Geometry: see drawing. Coordinates: mm, zero at the bounding-box minimum. A direction names the side the tool comes from. Give positions to 0.01 mm unless a question says otherwise; leave off trailing zeros. Write each loop counter-clockwise with the first axis right and the second up, starting at its lowest first coordinate (ties: lowest second). Pieces come first, ordered by that corner, then holes. Notation, with made-up numbers: (64, -7) - (79, -7) arc R12 cw to (79, -2) - close; hole circle Ø8 at (26, 41). An arc over 180 degrees is marked (long way). Return JSON: item names as keys, results as strings.
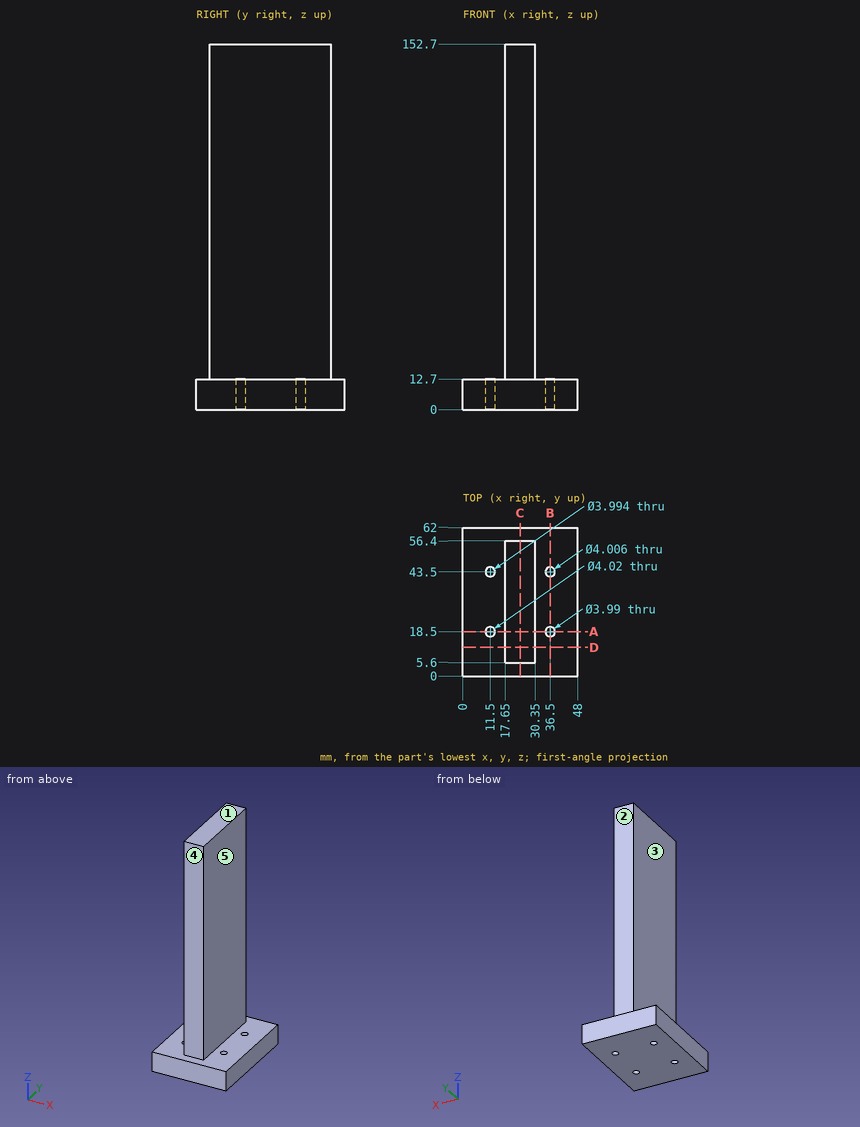
Q1. Set-up query: the marked faces 1, 2, 3, 4 and 5. Return all of +Z, -Z, +X, -X, +Y, -Y with unobstructed straight access to the full face (end or side cutting, diameter ignored); none if empty.
Answer key:
{"face 1": "+Z, +X, -X, +Y, -Y", "face 2": "+Z, +X, -X, +Y", "face 3": "+Z, -X, +Y, -Y", "face 4": "+Z, +X, -X, -Y", "face 5": "+Z, +X, +Y, -Y"}
Q2. Section query A-A, the plane y = 18.5. Count the separate pieces of the cut face and the enclosed holes in it, plus the area to 3 significant figures.
Answer key:
{"separate pieces": "3", "enclosed holes": "0", "area": "2,290 mm^2"}
Q3. Pin query (flat end, axial travel): P1, Ø3.5, axis at x = 11.5, y = 43.5, coming from the -Z side; P2, Ø8, axis at y = 49, z = 133.5, coming from the -X side; P3, Ø6, axis at x = 30, z = 23, coming from the -Y side; P4, Ø5, axis at x = 17.5, z = 115, coming from the +Y side. Return the tip coordinate at first contact, or that it passes through.
Answer key:
{"P1": "passes through", "P2": "stops at x = 17.65", "P3": "stops at y = 5.6", "P4": "stops at y = 56.4"}
Q4. Section query D-D, the plane y = 12. Return the cut outline in (x, z).
Answer key:
{"outline": "(0, 0) - (48, 0) - (48, 12.7) - (30.35, 12.7) - (30.35, 152.7) - (17.65, 152.7) - (17.65, 12.7) - (0, 12.7) - close"}
Q5. Material intervals for probe 1 along Y at (x, z) = (36.5, 9.5) (1 decimal); probe 2 along Y at (x, z) = (29.5, 120); probe 3 along Z at (x, y) = (4.5, 40.5), sorted ascending. Write a range as [from, to].
Answer key:
{"probe 1": "y = [0, 16.5], [20.5, 41.5], [45.5, 62]", "probe 2": "y = [5.6, 56.4]", "probe 3": "z = [0, 12.7]"}
Q6. Section query B-B, the plane x = 36.5. Return the cut outline in (y, z) (1 decimal), plus the area to 3 significant figures.
Answer key:
{"outline": "(0, 0) - (16.5, 0) - (16.5, 12.7) - (0, 12.7) - close; (20.5, 0) - (41.5, 0) - (41.5, 12.7) - (20.5, 12.7) - close; (45.5, 0) - (62, 0) - (62, 12.7) - (45.5, 12.7) - close", "area": "686 mm^2"}
Q7. Section query C-C, the plane x = 24. Return the cut outline in (y, z).
Answer key:
{"outline": "(0, 0) - (62, 0) - (62, 12.7) - (56.4, 12.7) - (56.4, 152.7) - (5.6, 152.7) - (5.6, 12.7) - (0, 12.7) - close"}
